Part print with two shaded views. Sizes in mm from the minimum x, y, z corner. A direction names the side the tool comes from. Round coordinates to 2 decimals unless told otherwise and drop trailing zeros. Write each loop counter-clockwise with the first axis right and the second up, starting at its lowest first coordinate (ties: lowest second). Pieces come first, ordered by that corner, then holes. Notation, with made-up numbers: (-12.75, -1.75) -> (24.25, -1.75) arc R16 ccw to (24.25, 26.25) -> close; hole circle Ø10 at (82, 43). An arc over 180 degrees is marked (long way). Answer as CSV lines item,"result".
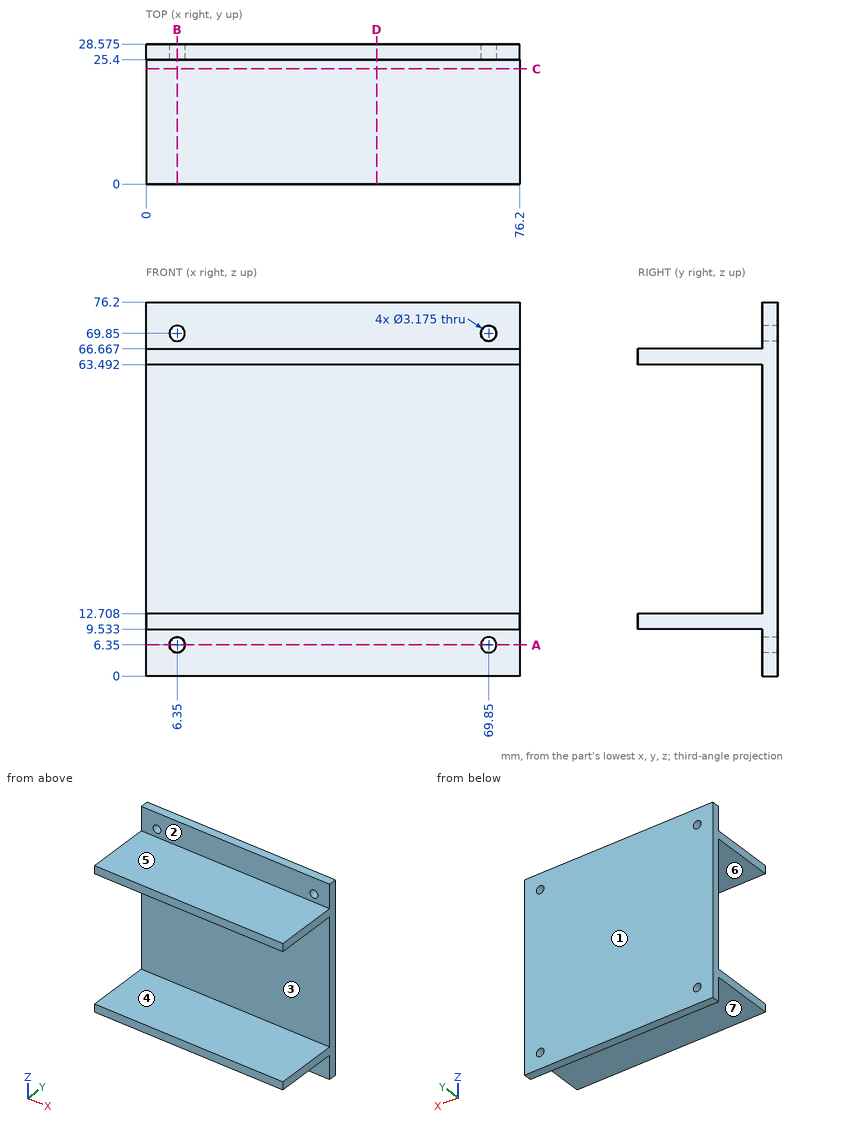
1. Mould opens along Z. For the marked faces 4, 5, 6 and 7 say: +Z half, -Z half, draft (parallel to the pull), parting line (faces both ways), or undercut.
Results found:
face 4,"undercut"
face 5,"+Z half"
face 6,"undercut"
face 7,"-Z half"
2. Which spindle directions (+Z, -Z, +X, -X, +Y, -Y) get a long thin tool onto all of the face, cutting with end or side? Do the marked faces 1, 2 and 3. Say none if no direction does.
Results found:
face 1,"+Z, -Z, +X, -X, +Y"
face 2,"+Z, +X, -X, -Y"
face 3,"+X, -X, -Y"
3. Probe line 1 along X through (y, z) = (26.8, 6.35); line 2 along Z through (x, y) = (44, 7.5). List the from-to ranges inside material, lowest first.
Results found:
line 1,"x = 0 to 4.76, 7.94 to 68.26, 71.44 to 76.2"
line 2,"z = 9.53 to 12.71, 63.49 to 66.67"
4. Cut at D-D, the plane x = 47. Write the cut outline in (y, z) (1 decimal).
Results found:
outline,"(0, 9.5) -> (25.4, 9.5) -> (25.4, 0) -> (28.6, 0) -> (28.6, 76.2) -> (25.4, 76.2) -> (25.4, 66.7) -> (0, 66.7) -> (0, 63.5) -> (25.4, 63.5) -> (25.4, 12.7) -> (0, 12.7) -> close"
5. Cut at C-C, the plane y = 23.5. Write the cut outline in (x, z), then the cut area to 3 significant figures.
Results found:
outline,"(0, 9.53) -> (76.2, 9.53) -> (76.2, 12.71) -> (0, 12.71) -> close; (0, 63.49) -> (76.2, 63.49) -> (76.2, 66.67) -> (0, 66.67) -> close"
area,"484 mm2"
6. Drop flat-ended pins along their axis: pin 1 Ø1.5 at (x, y) = (52, 11.5) entering from -Z; pin 2 Ø7.5 at (x, z) = (36.5, 5) entering from -Y; pin 3 Ø6 at (y, z) = (23.5, 37.5) entering from +X; pin 4 Ø12.5 at (x, y) = (35, 9.5) entering from +Z. Give the stop position or say it passes through.
Results found:
pin 1,"stops at z = 9.53"
pin 2,"stops at y = 25.4"
pin 3,"stops at x = 76.2"
pin 4,"stops at z = 66.67"
7. Cut at A-A, the plane z = 6.35. Write the cut outline in (x, y) (1 decimal).
Results found:
outline,"(0, 25.4) -> (4.8, 25.4) -> (4.8, 28.6) -> (0, 28.6) -> close; (7.9, 25.4) -> (68.3, 25.4) -> (68.3, 28.6) -> (7.9, 28.6) -> close; (71.4, 25.4) -> (76.2, 25.4) -> (76.2, 28.6) -> (71.4, 28.6) -> close"
8. Cut at B-B, the plane x = 6.35. Write the cut outline in (y, z) (1 decimal).
Results found:
outline,"(0, 9.5) -> (25.4, 9.5) -> (25.4, 7.9) -> (28.6, 7.9) -> (28.6, 68.3) -> (25.4, 68.3) -> (25.4, 66.7) -> (0, 66.7) -> (0, 63.5) -> (25.4, 63.5) -> (25.4, 12.7) -> (0, 12.7) -> close; (25.4, 0) -> (28.6, 0) -> (28.6, 4.8) -> (25.4, 4.8) -> close; (25.4, 71.4) -> (28.6, 71.4) -> (28.6, 76.2) -> (25.4, 76.2) -> close"
